from build123d import *

# Parameters (mm, degrees)
SKETCH_2_R      = 1
SKETCH_2_R_2    = 0.554445532
EXTRUDE_3_DEPTH = 0.75
SKETCH_2_5_R    = 1
EXTRUDE_4_DEPTH = 1.5
EXTRUDE_5_DEPTH = 0.75


with BuildPart() as part:
    # Sketch 2 → Extrude 3 (new body)
    # profile 1 of 2: a face of its own
    with BuildSketch(Plane(origin=(0, 0, 0), x_dir=(1, 0, 0), z_dir=(0, 1, 0))):
        with BuildLine():
            Line((-14.4, -3.425), (0, -3.425))
            ThreePointArc((0, -3.425), (3.425, 0), (0, 3.425))
            Line((0, 3.425), (-14.4, 3.425))
            ThreePointArc((-14.4, 3.425), (-17.825, 0), (-14.4, -3.425))
        make_face()
        with Locations(Location((-14.4, 0, 0), (0, 0, 270))):
            Circle(SKETCH_2_R, mode=Mode.SUBTRACT)
        with Locations(Location((0, 0, 0), (0, 0, 270))):
            Circle(SKETCH_2_R, mode=Mode.SUBTRACT)
    # profile 2 of 2: a face of its own
    with BuildSketch(Plane(origin=(0, 0, 0), x_dir=(1, 0, 0), z_dir=(0, 1, 0))):
        with BuildLine():
            ThreePointArc((-14.4, -3.425), (-14.550144339, -3.421707421), (-14.7, -3.411836016))
            Line((-14.7, -3.411836016), (-14.7, -7.575))
            Line((-14.7, -7.575), (0.3, -7.575))
            Line((0.3, -7.575), (0.3, -3.411836016))
            ThreePointArc((0.3, -3.411836016), (0.150144339, -3.421707421), (0, -3.425))
            Line((0, -3.425), (-14.4, -3.425))
        make_face()
        with Locations(Location((-13.55, -6.575, 0), (0, 0, 270))):
            Circle(SKETCH_2_R_2, mode=Mode.SUBTRACT)
        with Locations(Location((-11.01, -6.575, 0), (0, 0, 270))):
            Circle(SKETCH_2_R_2, mode=Mode.SUBTRACT)
        with Locations(Location((-8.47, -6.575, 0), (0, 0, 270))):
            Circle(SKETCH_2_R_2, mode=Mode.SUBTRACT)
        with Locations(Location((-5.93, -6.575, 0), (0, 0, 270))):
            Circle(SKETCH_2_R_2, mode=Mode.SUBTRACT)
        with Locations(Location((-3.39, -6.575, 0), (0, 0, 270))):
            Circle(SKETCH_2_R_2, mode=Mode.SUBTRACT)
        with Locations(Location((-0.85, -6.575, 0), (0, 0, 270))):
            Circle(SKETCH_2_R_2, mode=Mode.SUBTRACT)
    extrude(amount=EXTRUDE_3_DEPTH)

    # Sketch 2_5 → Extrude 4 (add)
    with BuildSketch(Plane(origin=(0, 0, 0), x_dir=(1, 0, 0), z_dir=(0, 1, 0))):
        with BuildLine():
            Line((0, 3.425), (-14.4, 3.425))
            ThreePointArc((-14.4, 3.425), (-17.821707421, 0.150144339), (-14.7, -3.411836016))
            ThreePointArc((-14.7, -3.411836016), (-14.550144339, -3.421707421), (-14.4, -3.425))
            Line((-14.4, -3.425), (0, -3.425))
            ThreePointArc((0, -3.425), (0.150144339, -3.421707421), (0.3, -3.411836016))
            ThreePointArc((0.3, -3.411836016), (3.421707421, 0.150144339), (0, 3.425))
        make_face()
        with Locations((-14.4, 0)):
            Circle(SKETCH_2_5_R, mode=Mode.SUBTRACT)
        Circle(SKETCH_2_5_R, mode=Mode.SUBTRACT)
    extrude(amount=EXTRUDE_4_DEPTH)

    # Sketch 3 → Extrude 5 (add)
    with BuildSketch(Plane(origin=(0, 1.5, 0), x_dir=(1, 0, 0), z_dir=(0, 1, 0))):
        with BuildLine():
            Line((-9.5, 2.5), (-4.9, 2.5))
            ThreePointArc((-4.9, 2.5), (-2.4, 0), (-4.9, -2.5))
            Line((-4.9, -2.5), (-9.5, -2.5))
            ThreePointArc((-9.5, -2.5), (-12, 0), (-9.5, 2.5))
        make_face()
    extrude(amount=EXTRUDE_5_DEPTH)


solid = part.part
Source: CAD feature listing. Evaluate the final solid. Frame: model axes, mm. A direction names the side the tool comes from. Coordinates: 2 decimals unless noted, no trailing zeros. Loops run counter-clockwise (first coordinate to the right, second up) from the corner with the lowest first, then second, coordinate; pieces in that order, holes last. Notation, with made-up numbers: (20, -36) - (33, -36) arc R26 cw to (33, -4) - close; hole circle Ø10 at (51.5, -10). An arc over 180 degrees is marked (long way). Return JSON: item names as keys, results as strings.
Q1. Section B-B, the plane x = -8.47. Return loops of the section in (y, z) (3 decimals).
Results:
{"outline": "(0, -3.425) - (1.5, -3.425) - (1.5, -2.5) - (2.25, -2.5) - (2.25, 2.5) - (1.5, 2.5) - (1.5, 3.425) - (0.75, 3.425) - (0.75, 6.021) - (0, 6.021) - close; (0, 7.129) - (0.75, 7.129) - (0.75, 7.575) - (0, 7.575) - close"}
Q2. Mould query, pull axis Z, two halves, no side actions, for faces 1 (the cylindrical face through (-12, 2, 0)), 2 (the flat face through (-7, 0.75, 5)), 3 (the flat face through (-7, 1, -3.425)), 4 (the cylindrical face through (-5.763, 0.37, 7.104)). Classes: released by +Z, released by -Z, zero draft, split by the parting line, or undercut.
Results:
{"face 1": "split by the parting line", "face 2": "zero draft", "face 3": "released by -Z", "face 4": "undercut"}
Q3. Contact query for flat-ended pins moving along their axis: P1, Ø4.5, axis at x = -5.5, z = 6, coming from the +Y side; P2, Ø0.8, axis at y = 0, z = 5.5, coming from the -X side; P3, Ø0.6, axis at y = 0, z = 5, coming from the +X side. Output: stop coordinate, or through.
Results:
{"P1": "y = 0.75", "P2": "x = -14.7", "P3": "x = 0.3"}
Q4. Material intervals for line 1 along X through (y, z) = (0.7, 0) (3 decimals); line 2 along Z through (x, y) = (-14.5, 1.05); line 3 along X through (y, z) = (0.5, 3.75), sorted ascending.
Results:
{"line 1": "-17.825 to -15.4, -13.4 to -1, 1 to 3.425", "line 2": "-3.42 to -0.99, 0.99 to 3.42", "line 3": "-14.7 to 0.3"}
Q5. Section C-C, the plane y = 0.95. Return loops of the section in (x, z) (3 decimals), plus the area to 3 significant figures.
Results:
{"outline": "(-14.4, -3.425) - (0, -3.425) arc R3.425 ccw to (0, 3.425) - (-14.4, 3.425) arc R3.425 ccw to start; hole circle Ø2 at (-14.4, 0); hole circle Ø2 at (0, 0)", "area": "129 mm2"}
Q6. Section A-A, the plane z = 0. Return loops of the section in (x, y) (3 decimals), plus the area to 3 significant figures.
Results:
{"outline": "(-17.825, 0) - (-15.4, 0) - (-15.4, 1.5) - (-17.825, 1.5) - close; (-13.4, 0) - (-1, 0) - (-1, 1.5) - (-2.4, 1.5) - (-2.4, 2.25) - (-12, 2.25) - (-12, 1.5) - (-13.4, 1.5) - close; (1, 0) - (3.425, 0) - (3.425, 1.5) - (1, 1.5) - close", "area": "33.1 mm2"}
Q7. Access query for faces 5 (the flat face through (-7, 1.5, 3)), 6 (the cylindrical face through (-13.383, 0.37, 7.104)), 7 (the cylindrical face through (-2.4, 1.9, -0.1)). Directions: +Z, -Z, +X, -X, +Y, -Y. A direction counts if a zero-diameter tool reaches every point of the face in a straight line with its end or side. Return the directions, or none.
Results:
{"face 5": "+Y", "face 6": "+Y, -Y", "face 7": "+X, +Y"}
Q8. Section D-D, the plane x = -0.5. Return loops of the section in (y, z) (3 decimals), plus the area to 3 significant figures.
Results:
{"outline": "(0, -3.425) - (1.5, -3.425) - (1.5, -0.866) - (0, -0.866) - close; (0, 0.866) - (1.5, 0.866) - (1.5, 3.425) - (0.75, 3.425) - (0.75, 6.145) - (0, 6.145) - close; (0, 7.005) - (0.75, 7.005) - (0.75, 7.575) - (0, 7.575) - close", "area": "10.1 mm2"}
